Source: CAD feature listing. Evaluate the final solid. Frame: model axes, mm. Round coordinates to 2 decimals unless told otherwise and drop trailing zeros. Loops run counter-clockwise (first coordinate to the right, second up) from the corner with the lowest first, then second, coordinate; pieces in that order, holes last.
Item 1: Section query B-B on x = -33. Return loops of the section in (y, z), then the cut area to 3 significant figures.
Item 2: Section query C-C on y = -70. Return loops of the section in (x, z).
Item 3: Section query A-A on y = -30. Return loops of the section in (x, z), then the cut area to 3 significant figures.
Item 4: First-contact query: P1, Ø3.5, axis at y = 8.5, z = -4, coming from the +X side; P2, Ø1.3, axis at y = -135, z = 5, coming from the -X side; P3, Ø10, axis at y = -79.5, z = 8.5, coming from the -X side; P4, Ø1.5, axis at x = -6.5, y = -41, coming from the -Z side. Flat tips, straight axial feed; report the tip coordinate or a pass-through.
Item 5: Section query D-D on z = 14.25. Return loops of the section in (x, y).
Item 6: Ray query, L1, parallel to Y at x = 32, z = 5; L2, parallel to Z at x = 25, y = -135; L3, parallel to Z at x = -28, y = -135. Return the intervals inside material, ascending.
```python
from build123d import *

# Parameters (mm, degrees)
SKETCH1_W           = 55
SKETCH1_H           = 10
BOSS_EXTRUDE1_DEPTH = 10
BOSS_EXTRUDE2_DEPTH = 10
SKETCH6_W           = 10
SKETCH6_H           = 10
BOSS_EXTRUDE3_DEPTH = 52
SKETCH7_W           = 57.683812306
SKETCH7_H           = 30
BOSS_EXTRUDE4_DEPTH = 3
SKETCH9_OUTSIDE_W   = 83.8
SKETCH9_OUTSIDE_H   = 203.8
SKETCH9_OUTSIDE_R   = 3
CUT_EXTRUDE1_DEPTH  = 35
SKETCH10_OUTSIDE_W  = 83.8
SKETCH10_OUTSIDE_H  = 203.8
SKETCH10_OUTSIDE_R  = 3
CUT_EXTRUDE2_DEPTH  = 35
BOSS_EXTRUDE6_REACH = 254.351
SKETCH14_R          = 3
SKETCH15_R          = 1.1
CUT_EXTRUDE3_DEPTH  = 230


with BuildPart() as part:
    # Sketch1 → Boss-Extrude1 (new body)
    with BuildSketch(Plane.XY):
        with Locations((27.5, 5)):
            Rectangle(SKETCH1_W, SKETCH1_H)
    extrude(amount=BOSS_EXTRUDE1_DEPTH)

    # Sketch3 → Boss-Extrude2 (add)
    with BuildSketch(Plane.XY.offset(10)):
        with BuildLine():
            Line((0, 0), (-18.993043386, -140))
            Line((-18.993043386, -140), (-31.688443832, -140))
            Line((-31.688443832, -140), (-11.238986316, 1.431015115))
            ThreePointArc((-11.238986316, 1.431015115), (-7.887509596, 7.56009759), (-1.341906153, 10))
            Line((-1.341906153, 10), (0, 10))
            Line((0, 10), (0, 0))
        make_face()
    boss_extrude2 = extrude(amount=-BOSS_EXTRUDE2_DEPTH)

    # Mirror1: Boss-Extrude2 across plane
    add(boss_extrude2.mirror(Plane(origin=(27.5, 0, 0), x_dir=(0, 0, 1), z_dir=(1, 0, 0))))

    # Sketch6 → Boss-Extrude3 (add)
    with BuildSketch(Plane(origin=(80, 0, 0), x_dir=(0, 0, -1), z_dir=(1, 0, 0))):
        with Locations((-5, -135)):
            Rectangle(SKETCH6_W, SKETCH6_H)
    boss_extrude3 = extrude(amount=BOSS_EXTRUDE3_DEPTH)

    # Mirror2: Boss-Extrude3 across plane
    add(boss_extrude3.mirror(Plane(origin=(27.5, 0, 0), x_dir=(0, 0, 1), z_dir=(1, 0, 0))))

    # Sketch7 → Boss-Extrude4 (add)
    with BuildSketch(Plane(origin=(0, 10, 0), x_dir=(1, 0, 0), z_dir=(0, 1, 0))):
        with Locations((27.5, -5)):
            Rectangle(SKETCH7_W, SKETCH7_H)
    extrude(amount=-BOSS_EXTRUDE4_DEPTH)

    # Sketch9 outside → Cut-Extrude1 (cut)
    with BuildSketch(Plane.ZY.offset(77)):
        with Locations((5, -65)):
            Rectangle(SKETCH9_OUTSIDE_W, SKETCH9_OUTSIDE_H)
        with Locations((5, -135)):
            Circle(SKETCH9_OUTSIDE_R, mode=Mode.SUBTRACT)
    extrude(amount=-CUT_EXTRUDE1_DEPTH, mode=Mode.SUBTRACT)

    # Sketch10 outside → Cut-Extrude2 (cut)
    with BuildSketch(Plane(origin=(132, 0, 0), x_dir=(0, 0, -1), z_dir=(1, 0, 0))):
        with Locations((-5, -65)):
            Rectangle(SKETCH10_OUTSIDE_W, SKETCH10_OUTSIDE_H)
        with Locations(Location((-5, -135, 0), (0, 0, 180))):
            Circle(SKETCH10_OUTSIDE_R, mode=Mode.SUBTRACT)
    extrude(amount=-CUT_EXTRUDE2_DEPTH, mode=Mode.SUBTRACT)

    # Boss-Extrude6: up to this plane
    boss_extrude6_end = Plane(origin=(0, 0, 0), z_dir=(-0.9909226687301317, 0.13443312313843575, 0))
    # Sketch14 → Boss-Extrude6 (add, up to the surface)
    with BuildSketch(Plane(origin=(132, 0, 0), x_dir=(0, 0, -1), z_dir=(1, 0, 0)), mode=Mode.PRIVATE) as boss_extrude6_sk1:
        with Locations(Location((-5, -135, 0), (0, 0, 180))):
            Circle(SKETCH14_R)
    boss_extrude6_tool1 = split(extrude(boss_extrude6_sk1.sketch, amount=-BOSS_EXTRUDE6_REACH, mode=Mode.PRIVATE), bisect_by=boss_extrude6_end, keep=Keep.BOTH, mode=Mode.PRIVATE)
    add(boss_extrude6_tool1.solids().sort_by_distance((132, -135, 5))[0])

    # Sketch15 → Cut-Extrude3 (cut)
    with BuildSketch(Plane.ZY.offset(77)):
        with Locations((5, -135)):
            Circle(SKETCH15_R)
    extrude(amount=-CUT_EXTRUDE3_DEPTH, mode=Mode.SUBTRACT)


solid = part.part
```
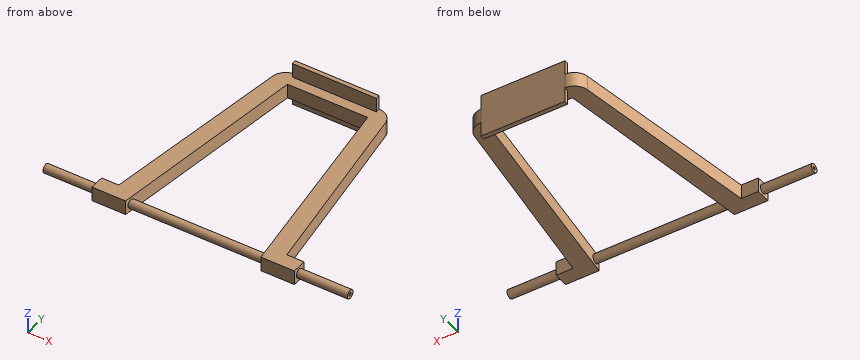
Data:
1. outline: (-140, 0) - (-130, 0) - (-130, 10) - (-140, 10) - close; hole circle Ø2.2 at (-135, 5)
1. area: 96.2 mm2
2. outline: (-21.57, 0) - (-9.5, 0) - (-9.5, 10) - (-21.57, 10) - close; (64.5, 0) - (76.57, 0) - (76.57, 10) - (64.5, 10) - close
3. outline: (-15.78, 0) - (-4.07, 0) - (-4.07, 10) - (-15.78, 10) - close; (59.07, 0) - (70.78, 0) - (70.78, 10) - (59.07, 10) - close
3. area: 234 mm2
4. P1: stops at x = 56.34
4. P2: passes through
4. P3: stops at x = -23.66
4. P4: stops at z = 0
5. outline: (-1.34, 7) - (56.34, 7) - (56.34, 10) - (-1.34, 10) - close
6. L1: y = -138 to -136.1, -133.9 to -132, 0 to 10
6. L2: z = 2 to 3.9, 6.1 to 8
6. L3: z = 0 to 3.9, 6.1 to 10
